Build history of the part. All positions in model axes, mm. A direction names the side the tool comes from. Coordinates: 2 decimals unless noted, no trailing zeros. Order: outer loops, then holes, each group sorted by start corner. A loop starts at its lowest first (then second) coordinate and runs counter-clockwise, first axis right, second up. Notation, with made-up numbers: (49, 84) - (98, 84) arc R15 cw to (98, 109) - close; hole circle Ø8 at (27, -16). An arc over 180 degrees is marked (long way). Return JSON: item names as keys, results as strings.
from build123d import *

# Parameters (mm, degrees)
SKETCH1_W               = 96.89
SKETCH1_H               = 90.17
PCB_DEPTH               = 1.57
SKETCH2_R               = 1.75
M3_MOUNTING_HOLES_DEPTH = 1.57
SKETCH4_R               = 1.75
CUT_EXTRUDE1_DEPTH      = 23
BOSS_EXTRUDE2_DEPTH     = 2
BOSS_EXTRUDE3_DEPTH     = 2
SKETCH9_W               = 3
SKETCH9_H               = 19
SKETCH9_W_2             = 7
CUT_EXTRUDE2_DEPTH      = 127.760011393
SKETCH10_W              = 0.5
SKETCH10_H              = 90.17
CUT_EXTRUDE3_DEPTH      = 10
SKETCH11_W              = 60
SKETCH11_H              = 60
CUT_EXTRUDE4_DEPTH      = 10


with BuildPart() as part:
    # Sketch1 → PCB (new body)
    with BuildSketch(Plane(origin=(0, 0, 0), x_dir=(1, 0, 0), z_dir=(0, 1, 0))):
        with Locations((16.200949951, 63.633996534)):
            Rectangle(SKETCH1_W, SKETCH1_H)
    extrude(amount=PCB_DEPTH)

    # Sketch2 → M3 Mounting Holes (cut)
    with BuildSketch(Plane(origin=(0, 1.57, 0), x_dir=(1, 0, 0), z_dir=(0, 1, 0))):
        with Locations(Location((58.565949951, 27.438996534, 0), (0, 0, 270))):
            Circle(SKETCH2_R)
        with Locations(Location((-27.164050049, 23.628996534, 0), (0, 0, 270))):
            Circle(SKETCH2_R)
        with Locations(Location((-27.164050049, 99.138996534, 0), (0, 0, 270))):
            Circle(SKETCH2_R)
        with Locations(Location((58.565949951, 101.098996534, 0), (0, 0, 270))):
            Circle(SKETCH2_R)
    extrude(amount=-M3_MOUNTING_HOLES_DEPTH, mode=Mode.SUBTRACT)

    # Sketch4 → Cut-Extrude1 (cut)
    with BuildSketch(Plane(origin=(0, 1.57, 0), x_dir=(1, 0, 0), z_dir=(0, 1, 0))):
        with Locations(Location((-20.894050049, 88.718996534, 0), (0, 0, 270))):
            Circle(SKETCH4_R)
        with Locations(Location((53.105949951, 88.718996534, 0), (0, 0, 270))):
            Circle(SKETCH4_R)
    extrude(amount=-CUT_EXTRUDE1_DEPTH, mode=Mode.SUBTRACT)

    # Sketch7 → Boss-Extrude2 (add)
    with BuildSketch(Plane.XY.offset(-46.718996534)):
        Polygon((27.755949951, 1.57), (19.438412086, 9.887537865), (16.073487816, 9.887537865), (7.755949951, 1.57), align=None)
    extrude(amount=BOSS_EXTRUDE2_DEPTH)

    # Sketch8 → Boss-Extrude3 (add)
    with BuildSketch(Plane.XY.offset(-108.718996534)):
        Polygon((27.755949951, 1.57), (19.438412086, 9.887537865), (16.073487816, 9.887537865), (7.755949951, 1.57), align=None)
    extrude(amount=BOSS_EXTRUDE3_DEPTH)

    # Sketch9 → Cut-Extrude2 (cut, through all)
    with BuildSketch(Plane(origin=(0, 1.57, 0), x_dir=(1, 0, 0), z_dir=(0, 1, 0))):
        with Locations((-10.744050049, 28.048996534)):
            Rectangle(SKETCH9_W, SKETCH9_H)
        with Locations((-3.744050049, 28.048996534)):
            Rectangle(SKETCH9_W_2, SKETCH9_H)
        with Locations((3.255949951, 28.048996534)):
            Rectangle(SKETCH9_W, SKETCH9_H)
    extrude(amount=-CUT_EXTRUDE2_DEPTH, mode=Mode.SUBTRACT)

    # Sketch10 → Cut-Extrude3 (cut)
    with BuildSketch(Plane(origin=(0, 1.57, 0), x_dir=(1, 0, 0), z_dir=(0, 1, 0))):
        with Locations((-31.994050049, 63.633996534)):
            Rectangle(SKETCH10_W, SKETCH10_H)
        with Locations((64.395949951, 63.633996534)):
            Rectangle(SKETCH10_W, SKETCH10_H)
    extrude(amount=-CUT_EXTRUDE3_DEPTH, mode=Mode.SUBTRACT)

    # Sketch11 → Cut-Extrude4 (cut)
    with BuildSketch(Plane(origin=(0, 1.57, 0), x_dir=(1, 0, 0), z_dir=(0, 1, 0))):
        with Locations((16.105949951, 76.718996534)):
            Rectangle(SKETCH11_W, SKETCH11_H)
    extrude(amount=-CUT_EXTRUDE4_DEPTH, mode=Mode.SUBTRACT)


solid = part.part
1. Drop flat-ended pins along their axis: pin 1 (4.5 mm diameter, centred on x = 58.57, z = -101.1, fed in from +Y); pin 2 (0.5 mm diameter, centred on x = -4, y = 1, fed in from +Z). Give the stop position or say it passes through.
Check values:
{"pin 1": "y = 1.57", "pin 2": "z = -37.55"}
2. Cut at C-C on z = -88.5. Give the cut face in (x, y).
Check values:
{"outline": "(-31.74, 0) - (-22.63, 0) - (-22.63, 1.57) - (-31.74, 1.57) - close; (-19.16, 0) - (-13.89, 0) - (-13.89, 1.57) - (-19.16, 1.57) - close; (46.11, 0) - (51.37, 0) - (51.37, 1.57) - (46.11, 1.57) - close; (54.84, 0) - (64.15, 0) - (64.15, 1.57) - (54.84, 1.57) - close"}
3. Mould opens along Z. For faces 3 (the flat face through (11.973, 5.787, -107.733)), 4 (the flat face through (18, 5, -44.719)), 5 (the flat face through (16, 2, -106.719)) say: pulls with the +Z half, pulls with the -Z half, needs draft (parallel to the pull), parting line crosses it, or undercut.
Check values:
{"face 3": "needs draft", "face 4": "pulls with the +Z half", "face 5": "undercut"}
4. Tool access for faces 1 (the flat face through (23.655, 5.671, -45.733)), 2 (the flat face through (16, 2, -46.719)): list every direction of +Z, -Z, +X, -X, +Y, -Y with a clear straight run to the whole face (end or side of a thin tool).
Check values:
{"face 1": "+Z, -Z, +X, +Y", "face 2": "+Y, -Y"}
5. Cut at A-A on z = -53.5. Give the cut face in (x, y).
Check values:
{"outline": "(-31.74, 0) - (-13.89, 0) - (-13.89, 1.57) - (-31.74, 1.57) - close; (46.11, 0) - (64.15, 0) - (64.15, 1.57) - (46.11, 1.57) - close"}
6. Probe L1, parallel to Z at x = -9.5, y = 1.5; L2, parallel to X at y = 1.5, z = -65; L3, parallel to Y at x = 58, z = -87. List the from-to ranges inside material, lowest first.
Check values:
{"L1": "-108.72 to -106.72, -46.72 to -37.55", "L2": "-31.74 to -13.89, 46.11 to 64.15", "L3": "0 to 1.57"}
7. Cut at B-B on x = 41. Give the cut face in (y, z).
Check values:
{"outline": "(0, -108.72) - (1.57, -108.72) - (1.57, -106.72) - (0, -106.72) - close; (0, -46.72) - (1.57, -46.72) - (1.57, -18.55) - (0, -18.55) - close"}
